Check sheet for the modelled part. Datum: model origin and axes. Units: mm. A direction names the side the tool comes from. Round coordinates to 2 decimals unless told otherwise and drop trailing zeros. Write each loop counter-clockwise with the first axis right and the second up, starting at its lowest first coordinate (ties: lowest second). Pieces come first, ordered by that corner, then holes. Notation, with made-up numbers: (-29, -11) -> (-25, -11) arc R21 cw to (-25, 3) -> close; hole circle Ø1 at (-34.5, 25). An arc over 180 degrees is marked (long way). One line per item, written item: value.
from build123d import *

# Parameters (mm, degrees)
F0_R     = 22.5
F1_DEPTH = 4
F0_R_2   = 21
F2_DEPTH = 25
F3_R     = 5
F4_R     = 0.5
F0_R_3   = 20
F5_DEPTH = 3


with BuildPart() as f1:
    # F0 (on Front) → F1 (new body)
    with BuildSketch(Plane.XZ):
        Polygon((40, 25), (-40, 25), (-40, 0), (-40, -25), (40, -25), (40, 0), align=None)
        with BuildLine():
            ThreePointArc((-27.25, -15), (-34.078427, -17.828427), (-31.25, -11))
            ThreePointArc((-31.25, -11), (-28.421573, -12.171573), (-27.25, -15))
        make_face(mode=Mode.SUBTRACT)
        with BuildLine():
            ThreePointArc((35.25, -15), (28.421573, -17.828427), (31.25, -11))
            ThreePointArc((31.25, -11), (34.078427, -12.171573), (35.25, -15))
        make_face(mode=Mode.SUBTRACT)
        with BuildLine():
            ThreePointArc((-27.25, 15), (-28.421573, 12.171573), (-31.25, 11))
            ThreePointArc((-31.25, 11), (-34.078427, 17.828427), (-27.25, 15))
        make_face(mode=Mode.SUBTRACT)
        Circle(F0_R, mode=Mode.SUBTRACT)
        with BuildLine():
            ThreePointArc((35.25, 15), (34.078427, 12.171573), (31.25, 11))
            ThreePointArc((31.25, 11), (28.421573, 17.828427), (35.25, 15))
        make_face(mode=Mode.SUBTRACT)
    extrude(amount=F1_DEPTH)

    # F0 (on Front) → F2 (join)
    with BuildSketch(Plane.XZ):
        Circle(F0_R)
        Circle(F0_R_2, mode=Mode.SUBTRACT)
    extrude(amount=F2_DEPTH)

    # F3
    f3_edges = [f1.edges().sort_by_distance(p)[0] for p in [
        (-40, -2, -25),
        (-40, -2, 25),
        (40, -2, 25),
        (40, -2, -25),
    ]]
    fillet(f3_edges, radius=F3_R)

    # F4
    f4_edges = [f1.edges().sort_by_distance(p)[0] for p in [
        (-22.5, -25, 0),
        (-21, -25, 0),
    ]]
    fillet(f4_edges, radius=F4_R)

    # F0 (on Front) → F5 (join)
    with BuildSketch(Plane.XZ):
        Circle(F0_R_2)
        Circle(F0_R_3, mode=Mode.SUBTRACT)
    extrude(amount=F5_DEPTH)


solid = f1.part
Item 1: Sectioned sample at A-A (x = 0). Enter the section's corners in (y, z), then the cut area to 3 significant figures.
Result set:
outline: (-25, -22) arc R0.5 ccw to (-24.5, -22.5) -> (-4, -22.5) -> (-4, -25) -> (0, -25) -> (0, -20) -> (-3, -20) -> (-3, -21) -> (-24.5, -21) arc R0.5 ccw to (-25, -21.5) -> close; (-25, 21.5) arc R0.5 ccw to (-24.5, 21) -> (-3, 21) -> (-3, 20) -> (0, 20) -> (0, 25) -> (-4, 25) -> (-4, 22.5) -> (-24.5, 22.5) arc R0.5 ccw to (-25, 22) -> close
area: 101 mm^2
Item 2: Sectioned sample at C-C (z = 13). State how many separate pieces and enclosed holes the cut face has, then the cut area to 3 significant figures.
Result set:
separate pieces: 4
enclosed holes: 0
area: 219 mm^2
Item 3: Material ranges on line 1 along Z through (x, y) = (-31.25, -0.9); line 2 along X through (y, z) = (-1.4, -15); line 3 along X through (y, z) = (-9.75, 9.5), recorded low to high.
Result set:
line 1: -25 to -19, -11 to 11, 19 to 25
line 2: -40 to -35.25, -27.25 to -13.23, 13.23 to 27.25, 35.25 to 40
line 3: -20.4 to -18.73, 18.73 to 20.4
Item 4: Release check for a two-part mould opening along Z. For faces 3 (the cylindrical face through (20.03, -13.6, 6.31)), 4 (the cylindrical face through (-38, -2, 24)), 5 (the cylindrical face through (-39, -2, -23)) record: pulls with the +Z half, pulls with the -Z half, needs draft (parallel to the pull), parting line crosses it, or undercut.
Result set:
face 3: undercut
face 4: pulls with the +Z half
face 5: pulls with the -Z half
Item 5: Tool access check on faces 1 (the cylindrical face through (38, -2, 24)), 2 (the cylindrical face through (10.382, -14.106, -19.961)). Record the directions out of +Z, -Z, +X, -X, +Y, -Y that give a thin tool (end or side, any length) a straight path to the whole face; none if there is none.
Result set:
face 1: +Z, +X, +Y, -Y
face 2: -Y
Item 6: Sectioned sample at B-B (y = -14). Enter the section's corners in (x, z), then the cut area to 3 significant figures.
Result set:
outline: circle Ø45 at (0, 0); hole circle Ø42 at (0, 0)
area: 205 mm^2
Item 7: Depth check by flat-ended pin: pin 1 (12.5 mm diameter, centred on x = 4, z = 9.5, fed in from -Y); pin 2 (13 mm diameter, centred on x = -31.25, z = -15, fed in from +Y); pin 3 (2 mm diameter, centred on y = -18, z = -8.5, fed in from -X); pin 4 (10.5 mm diameter, centred on x = 31.25, z = 15, fed in from -Y). Enter the tip coordinate at first touch or a pass-through.
Result set:
pin 1: through
pin 2: y = 0
pin 3: x = -21.21
pin 4: y = -4
